from build123d import *

# Parameters (mm, degrees)
EXTRUDE_1_DEPTH     = 20
SKETCH_2_R          = 3
CUT_EXTRUDE_1_DEPTH = 58.341084747
SKETCH_3_R          = 1.5
CUT_EXTRUDE_2_DEPTH = 56.398555938


with BuildPart() as part:
    # 草图1 → 凸台-拉伸1 (new body)
    with BuildSketch(Plane.XY):
        Polygon((0, 0), (0, 38), (3, 38), (3, 3), (38, 3), (38, 0), align=None)
    extrude(amount=EXTRUDE_1_DEPTH)

    # 草图2 → 切除-拉伸1 (cut, through all)
    with BuildSketch(Plane.ZY):
        with Locations((10, 20)):
            Circle(SKETCH_2_R)
    extrude(amount=-CUT_EXTRUDE_1_DEPTH, mode=Mode.SUBTRACT)

    # 草图3 → 切除-拉伸2 (cut, through all)
    with BuildSketch(Plane(origin=(0, 3, 0), x_dir=(1, 0, 0), z_dir=(0, 1, 0))):
        with Locations(Location((18, -4, 0), (0, 0, 270))):
            Circle(SKETCH_3_R)
        with Locations(Location((18, -16, 0), (0, 0, 270))):
            Circle(SKETCH_3_R)
        with Locations(Location((30, -4, 0), (0, 0, 270))):
            Circle(SKETCH_3_R)
        with Locations(Location((30, -16, 0), (0, 0, 270))):
            Circle(SKETCH_3_R)
    extrude(amount=-CUT_EXTRUDE_2_DEPTH, mode=Mode.SUBTRACT)


solid = part.part
Geometry check sheet. Reference: the model listing, model coordinates, mm. A direction names the side the tool comes from. Give positions to 0.01 mm unless a question says otherwise; leave off trailing zeros. Loops run counter-clockwise (first coordinate to the right, second up) from the corner with the lowest first, then second, coordinate; pieces in that order, holes last. Notation, with made-up numbers: (-0.75, 5.25) -> (48.25, 5.25) arc R15 cw to (48.25, 23.25) -> close; hole circle Ø11 at (-1, 42.25). An arc over 180 degrees is marked (long way). Answer in a Markdown table with one row per item. Add a question column.
1) Material ranges on probe 1 along X at (y, z) = (1.55, 4); probe 2 along Y at (x, z) = (1.7, 10); probe 3 along Y at (x, z) = (33.5, 6.25), recorded low to high. Write a range as from..to.
2) Cross-section at A-A on y = 20. Record the boundary of the cut face in (x, z), and give its area (3 significant figures).
3) Set-up check for faces 1 (the face through (20, 3, 10)), 2 (the face through (19.265, 1.521, 4.806)): record each of +Z, -Z, +X, -X, +Y, -Y from which the full face is reachable in a straight line by a thin tool's end or side.
4) Cross-section at C-C on z = 16. Record the boundary of the cut face in (x, y), and give its area (3 significant figures).
5) Cross-section at D-D on z = 9.25. Record the boundary of the cut face in (x, y), and give its area (3 significant figures).
6) Draft check along Y on faces 3 (the face through (19, 0, 10)), 4 (the face through (1.48, 18.85, 12.77)), 5 (the face through (3, 25, 10)). Enter one of: pulls with the +Y half, pulls with the -Y half, needs draft (parallel to the pull), parting line crosses it, or undercut.
7) Gauge pin test, flat ends, axial feed: P1, Ø6, axis at x = 22, z = 9, coming from the +Y side; P2, Ø10, axis at y = 28, z = 7.5, coming from the +X side; P3, Ø2.5, axis at x = 30, z = 16, coming from the -Y side. Record the tip position at first contact, or that the pin passes through.
8) Cross-section at B-B on x = 18. Record the boundary of the cut face in (y, z).
Outcome:
| question | item | result |
|---|---|---|
| 1 | probe 1 | x = 0..16.5, 19.5..28.5, 31.5..38 |
| 1 | probe 2 | y = 0..17, 23..38 |
| 1 | probe 3 | y = 0..3 |
| 2 | outline | (0, 0) -> (3, 0) -> (3, 7) -> (0, 7) -> close; (0, 13) -> (3, 13) -> (3, 20) -> (0, 20) -> close |
| 2 | area | 42.0 mm^2 |
| 3 | face 1 | +Z, -Z, +X, +Y |
| 3 | face 2 | +Y, -Y |
| 4 | outline | (0, 0) -> (16.5, 0) -> (16.5, 3) -> (3, 3) -> (3, 38) -> (0, 38) -> close; (19.5, 0) -> (28.5, 0) -> (28.5, 3) -> (19.5, 3) -> close; (31.5, 0) -> (38, 0) -> (38, 3) -> (31.5, 3) -> close |
| 4 | area | 201 mm^2 |
| 5 | outline | (0, 0) -> (38, 0) -> (38, 3) -> (3, 3) -> (3, 17.1) -> (0, 17.1) -> close; (0, 22.9) -> (3, 22.9) -> (3, 38) -> (0, 38) -> close |
| 5 | area | 202 mm^2 |
| 6 | face 3 | pulls with the -Y half |
| 6 | face 4 | undercut |
| 6 | face 5 | needs draft |
| 7 | P1 | stops at y = 3 |
| 7 | P2 | stops at x = 3 |
| 7 | P3 | passes through |
| 8 | outline | (0, 0) -> (3, 0) -> (3, 2.5) -> (0, 2.5) -> close; (0, 5.5) -> (3, 5.5) -> (3, 14.5) -> (0, 14.5) -> close; (0, 17.5) -> (3, 17.5) -> (3, 20) -> (0, 20) -> close |
